Verification items for the finished model (mm, model axes). Face numbers are marked on the shaded views. Round coordinates to 2 decimals unless told otherwise and drop trailing zeros. Write each loop counter-clockwise with the first axis right and the second up, starting at its lowest first coordinate (ties: lowest second). Pieces come first, ordered by that corner, then holes. Notation, with made-up numbers: (-24, 41) -> (34, 41) arc R20 cw to (34, 46) -> close; hole circle Ø11 at (-18, 58). An arc over 180 degrees is marked (long way). Use CSV: the item, a comma, the result in double quotes.
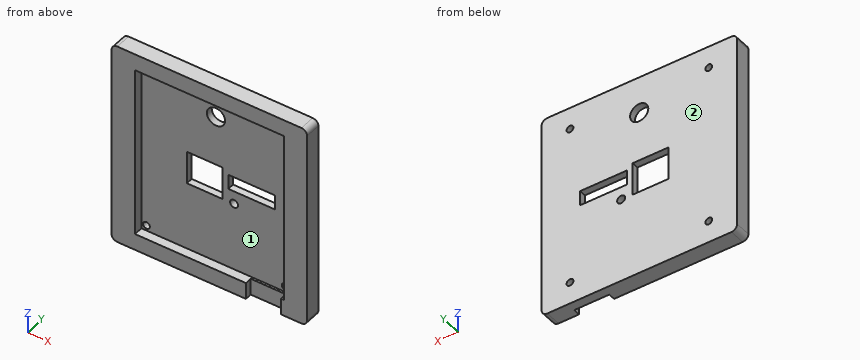
```python
from build123d import *

# Parameters (mm, degrees)
SKETCH_1_W           = 85.8
SKETCH_1_H           = 90
SKETCH_1_W_2         = 65.278
SKETCH_1_H_2         = 75.438
EXTRUDE_1_DEPTH      = 4
SKETCH_6_W           = 85.8
SKETCH_6_H           = 90
EXTRUDE_2_DEPTH      = 3
SKETCH_7_W           = 15.4
SKETCH_7_H           = 7.281
CUT_EXTRUDE_1_DEPTH  = 3
FILLET_1_R           = 2.5
CUT_EXTRUDE_2_DEPTH  = 118.835684599
SKETCH_10_R          = 1.75
CUT_EXTRUDE_3_DEPTH  = 118.835684599
SKETCH_11_W          = 15.621
SKETCH_11_H          = 14.5
CUT_EXTRUDE_4_DEPTH  = 118.835684599
SKETCH_15_R          = 4
CUT_EXTRUDE_8_DEPTH  = 118.835684599
SKETCH_12_R          = 1.5
CUT_EXTRUDE_15_DEPTH = 10


with BuildPart() as part:
    # 草图1 → 凸台-拉伸1 (new body)
    with BuildSketch(Plane(origin=(0, 0, 0), x_dir=(1, 0, 0), z_dir=(0, 1, 0))):
        with Locations((38.264980184, 40.138091102)):
            Rectangle(SKETCH_1_W, SKETCH_1_H)
        with Locations((38.264980184, 40.138091102)):
            Rectangle(SKETCH_1_W_2, SKETCH_1_H_2, mode=Mode.SUBTRACT)
    extrude(amount=EXTRUDE_1_DEPTH)

    # 草图6 → 凸台-拉伸2 (add)
    with BuildSketch(Plane(origin=(0, 4, 0), x_dir=(1, 0, 0), z_dir=(0, 1, 0))):
        with Locations((38.264980184, 40.138091102)):
            Rectangle(SKETCH_6_W, SKETCH_6_H)
    extrude(amount=EXTRUDE_2_DEPTH)

    # 草图7 → 切除-拉伸1 (cut)
    with BuildSketch(Plane.XZ):
        with Locations((61.997000004, -81.497591102)):
            Rectangle(SKETCH_7_W, SKETCH_7_H)
    extrude(amount=-CUT_EXTRUDE_1_DEPTH, mode=Mode.SUBTRACT)

    # 圆角1
    fillet_1_edges = [part.edges().sort_by_distance(p)[0] for p in [
        (-4.635019816, 3.5, -85.138091102),
        (81.164980184, 3.5, -85.138091102),
        (81.164980184, 3.5, 4.861908898),
        (-4.635019816, 3.5, 4.861908898),
    ]]
    fillet(fillet_1_edges, radius=FILLET_1_R)

    # 草图9 → 切除-拉伸2 (cut, through all)
    with BuildSketch(Plane(origin=(0, 7, 0), x_dir=(1, 0, 0), z_dir=(0, 1, 0))):
        Polygon((64.254980184, 41.998091102), (47.299239867, 41.998091102), (43.754980184, 41.998091102), (43.754980184, 35.498091102), (64.254980184, 35.498091102), align=None)
    extrude(amount=-CUT_EXTRUDE_2_DEPTH, mode=Mode.SUBTRACT)

    # 草图10 → 切除-拉伸3 (cut, through all)
    with BuildSketch(Plane(origin=(0, 7, 0), x_dir=(1, 0, 0), z_dir=(0, 1, 0))):
        with Locations(Location((46.264980184, 47.688091102, 0), (0, 0, 270))):
            Circle(SKETCH_10_R)
    extrude(amount=-CUT_EXTRUDE_3_DEPTH, mode=Mode.SUBTRACT)

    # 草图11 → 切除-拉伸4 (cut, through all)
    with BuildSketch(Plane(origin=(0, 7, 0), x_dir=(1, 0, 0), z_dir=(0, 1, 0))):
        with Locations((33.394480184, 40.588091102)):
            Rectangle(SKETCH_11_W, SKETCH_11_H)
    extrude(amount=-CUT_EXTRUDE_4_DEPTH, mode=Mode.SUBTRACT)

    # 草图15 → 切除-拉伸8 (cut, through all)
    with BuildSketch(Plane(origin=(0, 7, 0), x_dir=(1, 0, 0), z_dir=(0, 1, 0))):
        with Locations(Location((38.353887366, 11.356570823, 0), (0, 0, 270))):
            Circle(SKETCH_15_R)
    extrude(amount=-CUT_EXTRUDE_8_DEPTH, mode=Mode.SUBTRACT)

    # 草图12 → 切除-拉伸15 (cut)
    with BuildSketch(Plane(origin=(0, 7, 0), x_dir=(1, 0, 0), z_dir=(0, 1, 0))):
        with Locations(Location((7.825980184, 75.457091102, 0), (0, 0, 270))):
            Circle(SKETCH_12_R)
        with Locations(Location((68.703980184, 75.457091102, 0), (0, 0, 270))):
            Circle(SKETCH_12_R)
        with Locations(Location((7.825980184, 4.819091102, 0), (0, 0, 270))):
            Circle(SKETCH_12_R)
        with Locations(Location((68.703980184, 4.819091102, 0), (0, 0, 270))):
            Circle(SKETCH_12_R)
    extrude(amount=-CUT_EXTRUDE_15_DEPTH, mode=Mode.SUBTRACT)


solid = part.part
```
Q1. Section check C-C (y = 5.5). State how many separate pieces and enclosed holes the cut face has, plus the area to 3 significant figures.
Filled in:
separate pieces,"1"
enclosed holes,"8"
area,"7,270 mm²"
Q2. Section check B-B (z = -79.5). Record the cut outline in (x, y).
Filled in:
outline,"(-4.64, 0) -> (54.3, 0) -> (54.3, 3) -> (69.7, 3) -> (69.7, 0) -> (81.16, 0) -> (81.16, 7) -> (-4.64, 7) -> close"
Q3. Go/stop test with flat-tipped pins: P1, Ø5, axis at x = 7.83, z = -4.82, coming from the -Y side; P2, Ø10.5, axis at x = 38.35, z = -11.36, coming from the -Y side. Record where each tip stops, or that it passes through.
Filled in:
P1,"y = 0"
P2,"y = 4"
Q4. Section check A-A (x = 33). Record the cut outline in (y, z), plus the area to 3 significant figures.
Filled in:
outline,"(0, -85.14) -> (7, -85.14) -> (7, -47.84) -> (4, -47.84) -> (4, -77.86) -> (0, -77.86) -> close; (0, -2.42) -> (4, -2.42) -> (4, -33.34) -> (7, -33.34) -> (7, 4.86) -> (0, 4.86) -> close"
area,"285 mm²"
Q5. Mould release check, pull along Z, two halves, no side actions. Record for the marked faces 1 and 2: released by +Z, released by -Z, zero draft, split by the parting line, or undercut.
Filled in:
face 1,"undercut"
face 2,"zero draft"
Q6. Material ranges on L1, parallel to X at y = 2.25, z = -3.5; L2, parallel to Z at x = 59.5, y = 6.75; L3, parallel to Z at x = 40.5, y = 1.5, recorded low to high.
Filled in:
L1,"-4.64 to 5.63, 70.9 to 81.16"
L2,"-85.14 to -42, -35.5 to 4.86"
L3,"-85.14 to -77.86, -2.42 to 4.86"
Q7. Section check D-D (x = 57.5). Record the cut outline in (y, z).
Filled in:
outline,"(0, -2.42) -> (4, -2.42) -> (4, -35.5) -> (7, -35.5) -> (7, 4.86) -> (0, 4.86) -> close; (3, -85.14) -> (7, -85.14) -> (7, -42) -> (4, -42) -> (4, -77.86) -> (3, -77.86) -> close"
